Could you check a few things on this model? Use its own coordinates, in mm. A direction names the side the tool comes from. Round coordinates to 2 decimals unless told otherwise and drop trailing zeros. Write each loop counter-clockwise with the first axis right and the second up, starting at its lowest first coordinate (ties: lowest second). Pieces come first, ordered by that corner, then holes. Notation, with made-up numbers: (-4.75, 69) -> (11.25, 69) arc R16 cw to (11.25, 82) -> close; hole circle Ø5 at (-26.75, -9.5). An arc over 180 degrees is marked (long way). Answer in a Markdown table with one row per item.
from build123d import *

# Parameters (mm, degrees)
SKETCH1_R           = 10.725
BOSS_EXTRUDE1_DEPTH = 6
BOSS_EXTRUDE2_START = 6
SKETCH2_R           = 13
BOSS_EXTRUDE2_DEPTH = 2
BOSS_EXTRUDE3_START = -8
SKETCH2_2_R         = 13
BOSS_EXTRUDE3_DEPTH = 2
CUT_EXTRUDE1_REACH  = 26.372
SKETCH3_R           = 4


with BuildPart() as part:
    # Sketch1 → Boss-Extrude1 (new, symmetric)
    with BuildSketch(Plane(origin=(0, 0, 0), x_dir=(1, 0, 0), z_dir=(0, 1, 0))):
        with Locations(Location((0, 0, 0), (0, 0, 270))):
            Circle(SKETCH1_R)
    extrude(amount=BOSS_EXTRUDE1_DEPTH, both=True)

    # Sketch2 → Boss-Extrude2 (add)
    with BuildSketch(Plane(origin=(0, 0, 0), x_dir=(1, 0, 0), z_dir=(0, 1, 0)).offset(BOSS_EXTRUDE2_START)):
        with Locations(Location((0, 0, 0), (0, 0, 270))):
            Circle(SKETCH2_R)
    extrude(amount=BOSS_EXTRUDE2_DEPTH)

    # Sketch2<2> → Boss-Extrude3 (add)
    with BuildSketch(Plane(origin=(0, 0, 0), x_dir=(1, 0, 0), z_dir=(0, 1, 0)).offset(BOSS_EXTRUDE3_START)):
        with Locations(Location((0, 0, 0), (0, 0, 270))):
            Circle(SKETCH2_2_R)
    extrude(amount=BOSS_EXTRUDE3_DEPTH)

    # Sketch3 → Cut-Extrude1 (cut, up to next)
    with BuildSketch(Plane(origin=(0, 8, 0), x_dir=(1, 0, 0), z_dir=(0, 1, 0)), mode=Mode.PRIVATE) as cut_extrude1_sk1:
        with Locations(Location((0, 0, 0), (0, 0, 270))):
            Circle(SKETCH3_R)
    cut_extrude1_tool1 = extrude(cut_extrude1_sk1.sketch, amount=-CUT_EXTRUDE1_REACH, mode=Mode.PRIVATE) & part.part
    add(cut_extrude1_tool1.solids().sort_by_distance((0, 8, 0))[0], mode=Mode.SUBTRACT)


solid = part.part
1) For faces 1 (the face through (3.22, 0.08, 10.23)), 2 (the face through (-3.905, 0.112, -0.867)), which set-ups out of +Z, -Z, +X, -X, +Y, -Y let a thin tool reach every point of the face, with its end or its side?
Findings:
| item | result |
|---|---|
| face 1 | none |
| face 2 | +Y, -Y |
2) Imagine slicing it at C-C, the plane y = 7.25. Please give me the cut outline in (x, z).
Findings:
| item | result |
|---|---|
| outline | circle Ø26 at (0, 0); hole circle Ø8 at (0, 0) |
3) Thinking about a two-plate mould opening in Y: for faces 3 (the face through (11, -6, 2)), 4 (the face through (3, -8, 3)), 5 (the face through (11, 6, 2)), 6 (the face through (-7.91, -7.014, -10.316)), which applies, +Y half, -Y half, draft (parallel to the pull), parting line (faces both ways), or undercut?
Findings:
| item | result |
|---|---|
| face 3 | undercut |
| face 4 | -Y half |
| face 5 | undercut |
| face 6 | draft |
4) For pin 1 (6 mm diameter, centred on x = -7.5, y = -2, fed in from -Z); pin 2 (8 mm diameter, centred on y = -2.5, z = 4, fed in from +X); pin 3 (2 mm diameter, centred on x = 3.5, y = -6, fed in from +Z); pin 4 (6.5 mm diameter, centred on x = 0, z = 0, fed in from -Y), each with a flat end and sliding along its axis, tell me the tip position at first contact or that it passes through.
Findings:
| item | result |
|---|---|
| pin 1 | stops at z = -9.74 |
| pin 2 | stops at x = 12.84 |
| pin 3 | stops at z = 12.76 |
| pin 4 | passes through |
5) Please list where these lines run through material, in increasing order: line 1 (X direction, y = -4, z = 0) (3 decimals); line 2 (Y direction, x = -6.5, z = 9); line 3 (Z direction, x = 3, y = 4).
Findings:
| item | result |
|---|---|
| line 1 | x = -10.725 to -4, 4 to 10.725 |
| line 2 | y = -8 to -6, 6 to 8 |
| line 3 | z = -10.3 to -2.65, 2.65 to 10.3 |
6) Imagine slicing it at B-B, the plane z = 0. Please give me the cut outline in (x, y) (3 decimals).
Findings:
| item | result |
|---|---|
| outline | (-13, -8) -> (-4, -8) -> (-4, 8) -> (-13, 8) -> (-13, 6) -> (-10.725, 6) -> (-10.725, -6) -> (-13, -6) -> close; (4, -8) -> (13, -8) -> (13, -6) -> (10.725, -6) -> (10.725, 6) -> (13, 6) -> (13, 8) -> (4, 8) -> close |
7) Imagine slicing it at D-D, the plane z = 6.25. Please give me the cut outline in (x, y).
Findings:
| item | result |
|---|---|
| outline | (-11.4, -8) -> (11.4, -8) -> (11.4, -6) -> (8.72, -6) -> (8.72, 6) -> (11.4, 6) -> (11.4, 8) -> (-11.4, 8) -> (-11.4, 6) -> (-8.72, 6) -> (-8.72, -6) -> (-11.4, -6) -> close |
8) Imagine slicing it at A-A, the plane x = 0. Please give me the cut outline in (y, z) (3 decimals).
Findings:
| item | result |
|---|---|
| outline | (-8, -13) -> (-6, -13) -> (-6, -10.725) -> (6, -10.725) -> (6, -13) -> (8, -13) -> (8, -4) -> (-8, -4) -> close; (-8, 4) -> (8, 4) -> (8, 13) -> (6, 13) -> (6, 10.725) -> (-6, 10.725) -> (-6, 13) -> (-8, 13) -> close |
